Input: part model. Units: mm. Frame: model coordinates. Give positions to 0.01 mm unless a question says otherwise; leave off trailing zeros. Order: outer loops, then holes, each group sorted by start corner. A loop starts at its lowest first (then second) coordinate and runs counter-clockwise, first axis right, second up.
```python
from build123d import *

# Parameters (mm, degrees)
SKETCH_W   = 30
SKETCH_H   = 30
SKETCH_R   = 2
SKETCH_R_2 = 2.05
SKETCH_R_3 = 2.1
SKETCH_R_4 = 2.15
SKETCH_R_5 = 1.25
SKETCH_R_6 = 1.45
SKETCH_R_7 = 1.4
SKETCH_R_8 = 1.35
SKETCH_R_9 = 1.3
PAD_DEPTH  = 8


with BuildPart() as part:
    # Sketch → Pad (new body)
    with BuildSketch(Plane.XY):
        Rectangle(SKETCH_W, SKETCH_H)
        with Locations((-7.5, 10)):
            Circle(SKETCH_R, mode=Mode.SUBTRACT)
        with Locations((0, 10)):
            Circle(SKETCH_R_2, mode=Mode.SUBTRACT)
        with Locations((7.5, 10)):
            Circle(SKETCH_R_3, mode=Mode.SUBTRACT)
        with Locations((-7.5, 0)):
            Circle(SKETCH_R_4, mode=Mode.SUBTRACT)
        Circle(SKETCH_R_5, mode=Mode.SUBTRACT)
        with Locations((7.5, -10)):
            Circle(SKETCH_R_6, mode=Mode.SUBTRACT)
        with Locations((0, -10)):
            Circle(SKETCH_R_7, mode=Mode.SUBTRACT)
        with Locations((-7.5, -10)):
            Circle(SKETCH_R_8, mode=Mode.SUBTRACT)
        with Locations((7.5, 0)):
            Circle(SKETCH_R_9, mode=Mode.SUBTRACT)
    extrude(amount=PAD_DEPTH)


solid = part.part
```
1) Cut plane D-D (y = -1.75). Return the cut outline in (x, z), then the cut area to 3 significant figures.
2) Cut plane B-B (x = -7.5). Return the cut outline in (y, z), then the cut area to 3 significant figures.
3) Line query: probe 1 along Y at (x, z) = (-7.5, 4.75); probe 2 along Y at (x, z) = (7.5, 3.25); probe 3 along X at (y, z) = (0.5, 4). Output: solid intervals per line, ascending.
4) Cut plane C-C (z = 1.75). Count the separate pieces of the cut face and the enclosed holes in it, then the cut area to 3 significant figures.
5) Pull-direction query (X, two-part tool) for faces 1 (the face through (-8.974, 11.352, 3.944)), 2 (the face through (-15, 0, 4)), 3 (the face through (-4, 0, 8)); classes: pulls with the +X half, pulls with the -X half, needs draft (parallel to the pull), parting line crosses it, or undercut.
6) First-contact query: P1, Ø1.5, axis at x = 0, y = 0, coming from the -Z side; P2, Ø8, axis at x = -2, y = -8.5, coming from the -Z side. Flat tips, straight axial feed; report the tip coordinate or a pass-through.
7) Cut plane A-A (y = -10). Return the cut outline in (x, z), then the cut area to 3 significant figures.
Geometry says:
1. outline: (-15, 0) - (-8.75, 0) - (-8.75, 8) - (-15, 8) - close; (-6.25, 0) - (15, 0) - (15, 8) - (-6.25, 8) - close
1. area: 220 mm2
2. outline: (-15, 0) - (-11.35, 0) - (-11.35, 8) - (-15, 8) - close; (-8.65, 0) - (-2.15, 0) - (-2.15, 8) - (-8.65, 8) - close; (2.15, 0) - (8, 0) - (8, 8) - (2.15, 8) - close; (12, 0) - (15, 0) - (15, 8) - (12, 8) - close
2. area: 152 mm2
3. probe 1: y = -15 to -11.35, -8.65 to -2.15, 2.15 to 8, 12 to 15
3. probe 2: y = -15 to -11.45, -8.55 to -1.3, 1.3 to 7.9, 12.1 to 15
3. probe 3: x = -15 to -9.59, -5.41 to -1.15, 1.15 to 6.3, 8.7 to 15
4. separate pieces: 1
4. enclosed holes: 9
4. area: 817 mm2
5. face 1: undercut
5. face 2: pulls with the -X half
5. face 3: needs draft
6. P1: passes through
6. P2: stops at z = 0
7. outline: (-15, 0) - (-8.85, 0) - (-8.85, 8) - (-15, 8) - close; (-6.15, 0) - (-1.4, 0) - (-1.4, 8) - (-6.15, 8) - close; (1.4, 0) - (6.05, 0) - (6.05, 8) - (1.4, 8) - close; (8.95, 0) - (15, 0) - (15, 8) - (8.95, 8) - close
7. area: 173 mm2
